Part model, mm, in its own coordinate system. Face numbers are marked on the shaded views. Give positions to 0.01 mm unless a question says otherwise; leave off trailing zeros. Write each loop counter-clockwise with the first axis right and the second up, starting at its lowest first coordinate (ties: lowest second). Pieces come first, ordered by that corner, then holes. Notation, with made-up numbers: (57.5, 58.25) - (90.5, 58.25) arc R10 ccw to (90.5, 77.25) - close; hole circle Ø10 at (0.25, -34). An arc over 180 degrees is marked (long way). Answer in a Markdown table with one row per item. Add a question column.
1. Band-saw the part on C-C on x = 13. Write the cut outline in (y, z), plus the area to 3 significant figures.
2. Pull direction Z, two halves, no side cores. Call the marked faces 1, 2, 3 and 4: released by +Z, released by -Z, zero draft, split by the parting line, or undercut.
3. Band-saw the part on B-B on y = 0.3. Write the cut outline in (x, z).
4. Probe line 1 along X through (y, z) = (0.45, -5); line 2 along X through (y, z) = (0.3, -6.5); line 3 along Z through (x, y) = (12, 0.7). List the from-to ranges inside material, lowest first.
5. Drop a flat-ended pin along its axis: pin 1 Ø3 at (x, z) = (13, -5) entering from +Y. Give the stop position or say it passes through.
6. Band-saw the part on A-A on z = -5. Write the cut outline in (x, y), plus the area to 3 significant figures.
```python
from build123d import *

# Parameters (mm, degrees)
SKETCH1_W           = 26
SKETCH1_H           = 10
SKETCH1_R           = 2
BOSS_EXTRUDE1_DEPTH = 2
FILLET1_R           = 2


with BuildPart() as part:
    # Sketch1 → Boss-Extrude1 (new body)
    with BuildSketch(Plane(origin=(0, 0, 0), x_dir=(1, 0, 0), z_dir=(0, 1, 0))):
        with Locations((13, 5)):
            Rectangle(SKETCH1_W, SKETCH1_H)
        with Locations(Location((13, 5, 0), (0, 0, 270))):
            Circle(SKETCH1_R, mode=Mode.SUBTRACT)
    extrude(amount=BOSS_EXTRUDE1_DEPTH)

    # Fillet1
    fillet1_edges = [part.edges().sort_by_distance(p)[0] for p in [
        (0, 1, -10),
        (26, 1, -10),
        (26, 1, 0),
        (0, 1, 0),
    ]]
    fillet(fillet1_edges, radius=FILLET1_R)


solid = part.part
```
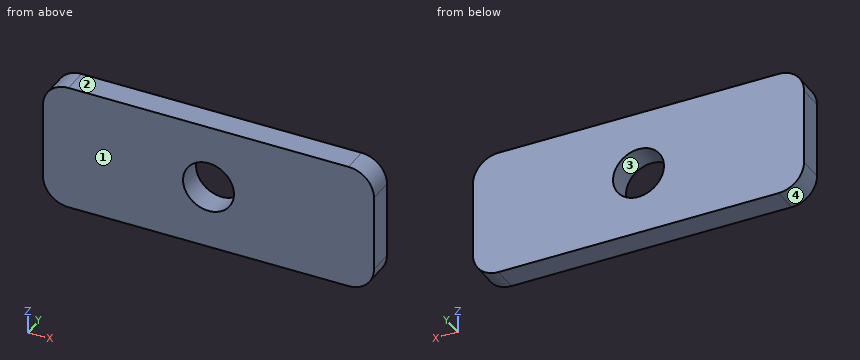
Values:
| question | item | result |
|---|---|---|
| 1 | outline | (0, -10) - (2, -10) - (2, -7) - (0, -7) - close; (0, -3) - (2, -3) - (2, 0) - (0, 0) - close |
| 1 | area | 12.0 mm² |
| 2 | face 1 | zero draft |
| 2 | face 2 | released by +Z |
| 2 | face 3 | undercut |
| 2 | face 4 | released by -Z |
| 3 | outline | (0, -8) arc R2 ccw to (2, -10) - (24, -10) arc R2 ccw to (26, -8) - (26, -2) arc R2 ccw to (24, 0) - (2, 0) arc R2 ccw to (0, -2) - close; hole circle Ø4 at (13, -5) |
| 4 | line 1 | x = 0 to 11, 15 to 26 |
| 4 | line 2 | x = 0 to 11.68, 14.32 to 26 |
| 4 | line 3 | z = -10 to -6.73, -3.27 to 0 |
| 5 | pin 1 | passes through |
| 6 | outline | (0, 0) - (11, 0) - (11, 2) - (0, 2) - close; (15, 0) - (26, 0) - (26, 2) - (15, 2) - close |
| 6 | area | 44.0 mm² |
